Autodesk Inventor part; units mm, degrees
ref_plane "YZ Plane" through (0, 0, 0) normal (1, 0, 0) x (0, 1, 0)
ref_plane "XZ Plane" through (0, 0, 0) normal (0, 1, 0) x (-1, 0, 0)
ref_plane "XY Plane" through (0, 0, 0) normal (0, 0, 1) x (1, 0, 0)
sketch "Sketch1" plane through (0, 0, 0) normal (0, 0, 1) x (1, 0, 0)
  line L0 (0, 0) -> (0, -25.4)
  line L1 (0, -25.4) -> (50.8, -25.4)
  line L2 (50.8, -25.4) -> (50.8, 0)
  line L3 (50.8, 0) -> (0, 0)
  line L4 (0, -25.4) -> (1.524, -25.4)
  line L5 (3.048, -22.352) -> (47.752, -22.352)
  line L6 (50.8, -25.4) -> (23.876, -25.4)
  line L7 (47.752, -22.352) -> (47.752, -3.048)
  line L8 (50.8, 0) -> (50.8, -1.524)
  line L9 (47.752, -3.048) -> (3.048, -3.048)
  line L10 (0, 0) -> (1.524, 0)
  line L11 (3.048, -22.352) -> (3.048, -3.048)
  dimension "d53" = 25.4
  dimension "d54" = 50.8
  dimension "d55" = 3.048
  dimension "d56" = 3.048
  dimension "d57" = 3.048
  dimension "d58" = 3.048
extrude "Extrusion1" add sketch "Sketch1" along normal blind 812.8
sketch "Sketch2" plane through (50.8, -25.4, 0) normal (1, 0, 0) x (0, 0, -1)
  line L0 (-812.8, 25.4) -> (-812.8, 0)
  line L1 (-812.8, 25.4) -> (-863.6, 25.4)
  line L2 (-863.6, 25.4) -> (-863.6, 0)
  line L3 (-863.6, 0) -> (-812.8, 0)
  line L4 (0, 0) -> (-812.8, 0)
  line L5 (-812.8, 25.4) -> (-812.8, 0)
  line L6 (-812.8, 0) -> (-815.848, 0)
  line L7 (-815.848, 3.048) -> (-815.848, 47.752)
  line L8 (-812.8, 25.4) -> (-812.8, 22.352)
  line L9 (-815.848, 47.752) -> (-860.552, 47.752)
  line L10 (-863.6, 25.4) -> (-860.552, 25.4)
  line L11 (-863.6, 0) -> (-863.6, 3.048)
  line L12 (-860.552, 3.048) -> (-815.848, 3.048)
  line L13 (-860.552, 47.752) -> (-860.552, 3.048)
  point P0 (0, 25.4)
extrude "Extrusion2" add sketch "Sketch2" against normal blind 254 contours L0 L3 L2 L1 L13 L12 L7 | L7 L12 L13 L1
sketch "Sketch3" plane through (0, -25.4, 0) normal (0, -1, 0) x (1, 0, 0)
  line L0 (0, 0) -> (50.8, 0)
  line L1 (50.8, 0) -> (0, 0)
  circle A0 centre (25.4, 25.4) radius 7.62
  circle A1 centre (25.4, 38.4302) radius 1.5875
  circle A2 centre (14.1155, 18.8849) radius 1.5875
  circle A3 centre (36.6845, 18.8849) radius 1.5875
  dimension "d23" = 360
extrude "Extrusion3" cut sketch "Sketch3" against normal blind 254
sketch "Sketch12" plane through (0, -25.4, 812.8) normal (0, 0, -1) x (-1, 0, 0)
  circle A0 centre (190.5, 6.35) radius 2.54
  line L0 (0, 25.4) -> (203.2, 25.4)
  line L1 (203.2, 25.4) -> (203.2, 0)
  dimension "d70" = 5.08
  dimension "d71" = 19.05
  dimension "d72" = 12.7
extrude "Extrusion10" cut sketch "Sketch12" against normal through all
sketch "Sketch13" plane through (0, -25.4, 0) normal (0, -1, 0) x (1, 0, 0)
  line L0 (50.8, 431.7892) -> (3.048, 431.7892)
  line L1 (0, 431.7892) -> (50.8, 431.7892)
  line L2 (50.8, 431.7892) -> (50.8, 457.1892)
  line L3 (50.8, 457.1892) -> (0, 457.1892)
  line L4 (0, 457.1892) -> (0, 431.7892)
  point P0 (50.8, 0)
sketch "Sketch14" plane through (0, 0, 0) normal (0, 1, 0) x (1, 0, 0)
  line L0 (50.8, -431.8) -> (0, -431.8)
  line L1 (50.8, -431.8) -> (50.8, -457.2)
  line L2 (50.8, -457.2) -> (0, -457.2)
  line L3 (0, -457.2) -> (0, -431.8)
  dimension "d78" = 25.4
properties part number "arm2v2" material "Aluminum 6061"
Check sheet for the modelled part. Datum: model origin and axes. Units: mm. A direction names the side the tool comes from. Round coordinates to 2 decimals unless told otherwise and drop trailing zeros. Loops run counter-clockwise (first coordinate to the right, second up) from the corner with the lowest first, then second, coordinate; pieces in that order, holes last. Notation, with made-up numbers: M -21,1 L 36,1 A15 cw 36,26 Z; hole C 87,-15.75 d7. An arc over 180 degrees is marked long. One line per question, with ' | ' between items. Start each with the question number.
Item 1: Scan lines: probe 1 along Y at (x, z) = (-190.5, 823.5); probe 2 along Y at (x, z) = (13.5, 478.5); probe 3 along X at (y, z) = (-3.75, 811.5). Record each from-to range of solid material in increasing order.
Item 2: Release check for a two-part mould opening along X. For faces 4 (the face through (-203.2, -13, 839)), 5 (the face through (-100, -13, 812.8)), 6 (the face through (26, -3.048, 401)) record: released by +X, released by -X, zero draft, split by the parting line, or undercut.
Item 3: Section check A-A (z = 540.5). Record the boundary of the cut face in (x, y).
Item 4: Gauge pin test, flat ends, axial feed: pin 1 Ø3.5 at (x, z) = (25.4, 38.43) entering from -Y; pin 2 Ø7.5 at (y, z) = (-9.5, 223) entering from -X; pin 3 Ø2 at (x, y) = (-49.5, -8.5) entering from -Z. Record the tip position at first contact, or that the pin passes through.
Item 5: Set-up check for faces 1 (the face through (0, -13, 401)), 2 (the face through (3.048, -13, 401)), 3 (the face through (-74, -13, 863.6)): record each of +Z, -Z, +X, -X, +Y, -Y from which the full face is reachable in a straight line by a thin tool's end or side.
Item 6: Section check B-B (y = -9). Record the boundary of the cut face in (x, z).
Item 7: Section check C-C (x = -84). Record the boundary of the cut face in (y, z), and give its area (3 significant figures).
Worked out:
1) probe 1: -25.4 to -21.59, -16.51 to 0 | probe 2: -25.4 to -22.35, -3.05 to 0 | probe 3: 0 to 3.05, 47.75 to 50.8
2) face 4: released by -X | face 5: zero draft | face 6: undercut
3) outline: M 0,-25.4 L 50.8,-25.4 L 50.8,0 L 0,0 Z; hole M 3.05,-22.35 L 47.75,-22.35 L 47.75,-3.05 L 3.05,-3.05 Z
4) pin 1: y = -25.4 | pin 2: x = 0 | pin 3: z = 812.8
5) face 1: -Z, -X, +Y, -Y | face 2: -Z | face 3: +Z, +X, -X, +Y, -Y
6) outline: M -203.2,812.8 L 0,812.8 L 0,0 L 3.05,0 L 3.05,812.8 L 47.75,812.8 L 47.75,0 L 50.8,0 L 50.8,863.6 L -203.2,863.6 Z
7) outline: M -25.4,812.8 L 0,812.8 L 0,863.6 L -25.4,863.6 Z | area: 1,290 mm^2
